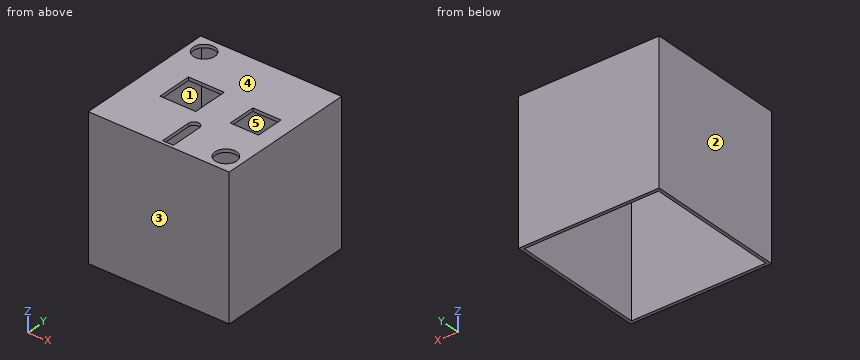
Solid Edge part; units mm, degrees
sketch "Sketch1" plane through (0, 0, 0) normal (0, 0, 1) x (1, 0, 0)
  line L0 (-65, 65) -> (-65, -65)
  line L1 (-65, -65) -> (65, -65)
  line L2 (65, -65) -> (65, 65)
  line L3 (65, 65) -> (-65, 65)
extrude "Protrusion1" add sketch "Sketch1" along normal blind 130
shell "Thinwall_1" thickness 3 removed faces 1 at (-44.6333, -42.0333, 0)
sketch "Sketch2" plane through (0, 0, 130) normal (0, 0, 1) x (0, 1, 0)
  line L0 (-16.5, 37.6302) -> (-16.5, 4.6302)
  line L1 (-16.5, 4.6302) -> (16.5, 4.6302)
  line L2 (16.5, 4.6302) -> (16.5, 37.6302)
  line L3 (16.5, 37.6302) -> (-16.5, 37.6302)
  circle A0 centre (50, 50) radius 10
  line L4 (-62, -11.0997) -> (-32, -11.0997)
  line L5 (-32, -1.0997) -> (-62, -1.0997)
  line L6 (-62, -1.0997) -> (-62, -11.0997)
  arc A1 (-32, -1.0997) -> (-32, -11.0997) centre (-32, -6.0997) cw
  circle A2 centre (-50, -50) radius 10
  line L7 (-13, -24.56) -> (-13, -50.56)
  line L8 (-13, -50.56) -> (13, -50.56)
  line L9 (13, -50.56) -> (13, -24.56)
  line L10 (13, -24.56) -> (-13, -24.56)
extrude "Cutout1" cut sketch "Sketch2" against normal up to next
Verification items for the finished model (mm, model axes). Face numbers are marked on the shaded views. A direction names the side the tool comes from. Round coordinates to 2 decimals unless told otherwise and drop trailing zeros. Loops run counter-clockwise (first coordinate to the right, second up) from the corner with the lowest first, then second, coordinate; pieces in that order, holes last. Notation, with made-up numbers: (82, 37.5) - (134, 37.5) arc R20 cw to (134, 62.5) - close; hole circle Ø9 at (50.25, 68.5). An arc over 180 degrees is marked (long way). Answer in a Markdown table with one row per item. Add a question column.
Q1. Section check C-C on z = 66. Enter the section's corners in (x, y).
Q2. Section check B-B on y = 50. Enter the section's corners in (x, z).
Q3. Material ranges on line 1 (X direction, y = -50, z = 129); line 2 (X direction, y = -0.5, z = 80.5); line 3 (Y direction, x = -50, z = 128.25), recorded low to high.
Q4. Section check A-A on x = 32.5. Enter the section's corners in (y, z), plus the area to 3 significant figures.
Q5. Gauge pin test, flat ends, axial feed: pin 1 (8 mm diameter, centred on x = 12, y = -2, fed in from -Z); pin 2 (23 mm diameter, centred on x = 50, y = -50, fed in from +Z). Record the tip position at first contact, or that the pin passes through.
Q6. Tool access check on the marked faces 4 and 5. Record the directions out of +Z, -Z, +X, -X, +Y, -Y that give a thin tool (end or side, any length) a straight path to the whole face; none if there is none.
Q7. Section check D-D on y = -50. Enter the section's corners in (x, z), plus the area to 3 significant figures.
Q8. Release check for a two-part mould opening along X. For the marked faces 1, 2 and 3 record: pulls with the +X half, pulls with the -X half, needs draft (parallel to the pull), parting line crosses it, or undercut.
Found:
| question | item | result |
|---|---|---|
| 1 | outline | (-65, -65) - (65, -65) - (65, 65) - (-65, 65) - close; hole (-62, -62) - (62, -62) - (62, 62) - (-62, 62) - close |
| 2 | outline | (-65, 0) - (-62, 0) - (-62, 127) - (-60, 127) - (-60, 130) - (-65, 130) - close; (-40, 127) - (62, 127) - (62, 0) - (65, 0) - (65, 130) - (-40, 130) - close |
| 3 | line 1 | x = -65 to 1.1, 11.1 to 40, 60 to 65 |
| 3 | line 2 | x = -65 to -62, 62 to 65 |
| 3 | line 3 | y = -65 to 40, 60 to 65 |
| 4 | outline | (-65, 0) - (-62, 0) - (-62, 127) - (-13, 127) - (-13, 130) - (-65, 130) - close; (13, 127) - (62, 127) - (62, 0) - (65, 0) - (65, 130) - (13, 130) - close |
| 4 | area | 1,070 mm² |
| 5 | pin 1 | stops at z = 127 |
| 5 | pin 2 | stops at z = 130 |
| 6 | face 4 | +Z, +X, -X, +Y, -Y |
| 6 | face 5 | -Z |
| 7 | outline | (-65, 0) - (-62, 0) - (-62, 127) - (1.1, 127) - (1.1, 130) - (-65, 130) - close; (11.1, 127) - (40, 127) - (40, 130) - (11.1, 130) - close; (60, 127) - (62, 127) - (62, 0) - (65, 0) - (65, 130) - (60, 130) - close |
| 7 | area | 1,060 mm² |
| 8 | face 1 | undercut |
| 8 | face 2 | pulls with the -X half |
| 8 | face 3 | needs draft |
